```python
from build123d import *

# Parameters (mm, degrees)
F1_DEPTH = 500


with BuildPart() as f1:
    # F0 (on Front) → F1 (new body, symmetric)
    with BuildSketch(Plane.XZ):
        Polygon((100, 100), (0, 100), (-100, 100), (-100, 75), (-25, 75), (-25, 0), (-25, -75), (-100, -75), (-100, -100), (0, -100), (100, -100), (100, -75), (25, -75), (25, 0), (25, 75), (100, 75), align=None)
    extrude(amount=F1_DEPTH, both=True)


solid = f1.part
```
Model file for the job. Use its own axes, mm. A direction names the side the tool comes from. Give positions to 0.01 mm unless a question says otherwise; leave off trailing zeros. Loops run counter-clockwise (first coordinate to the right, second up) from the corner with the lowest first, then second, coordinate; pieces in that order, holes last. Notation, with made-up numbers: (-4.5, 70) -> (41.5, 70) arc R17 cw to (41.5, 82) -> close; hole circle Ø5 at (72, -38.75). An arc over 180 degrees is marked (long way). Write each question's results on one line, items separated by ' | '.
(1) Pull direction Z, two halves, no side cores. Call faces 4 (the flat face through (63, -7, -75)), 5 (the flat face through (1, -7, 100)), 6 (the flat face through (-100, -7, -87)), 7 (the flat face through (-25, -7, 1)): released by +Z, released by -Z, zero draft, split by the parting line, or undercut.
Geometry results:
face 4: undercut | face 5: released by +Z | face 6: zero draft | face 7: undercut
(2) Flat gauge pins, fed straight in: pin 1 Ø10 at (y, z) = (78.5, 68.5) entering from -X; pin 2 Ø2 at (y, z) = (-105, 4) entering from +X. Where does each tip first touch, or does it go through?
Geometry results:
pin 1: stops at x = -25 | pin 2: stops at x = 25
(3) Tool access for faces 1 (the flat face through (-63, -7, 75)), 2 (the flat face through (100, -7, 87)), 3 (the flat face through (62, -7, 75)): list every direction of +Z, -Z, +X, -X, +Y, -Y with a clear straight run to the whole face (end or side of a thin tool).
Geometry results:
face 1: -X, +Y, -Y | face 2: +Z, -Z, +X, +Y, -Y | face 3: +X, +Y, -Y
(4) Cut at C-C on z = 49.5. List the corners of the cut face in (x, y).
Geometry results:
outline: (-25, -500) -> (25, -500) -> (25, 500) -> (-25, 500) -> close
(5) Probe line 1 along Z through (x, y) = (72, -369.5); line 2 along X through (y, z) = (-186.5, 57.5). List the from-to ranges inside material, lowest first.
Geometry results:
line 1: z = -100 to -75, 75 to 100 | line 2: x = -25 to 25
(6) Cut at A-A on x = -47. List the corners of the cut face in (y, z), and give its area (3 significant figures).
Geometry results:
outline: (-500, -100) -> (500, -100) -> (500, -75) -> (-500, -75) -> close; (-500, 75) -> (500, 75) -> (500, 100) -> (-500, 100) -> close | area: 50,000 mm²
(7) Cut at B-B on y = -210. List the corners of the cut face in (x, z), and give its area (3 significant figures).
Geometry results:
outline: (-100, -100) -> (100, -100) -> (100, -75) -> (25, -75) -> (25, 75) -> (100, 75) -> (100, 100) -> (-100, 100) -> (-100, 75) -> (-25, 75) -> (-25, -75) -> (-100, -75) -> close | area: 17,500 mm²
